from build123d import *

# Parameters (mm, degrees)
SKETCH_1_R          = 1.6
EXTRUDE_1_DEPTH     = 3
CUT_EXTRUDE_1_DEPTH = 85.905830189
FILLET_1_R          = 3
FILLET_2_R          = 10


with BuildPart() as part:
    # 草图1 → 凸台-拉伸1 (new body)
    with BuildSketch(Plane.XY):
        Polygon((0, 0), (20, 0), (60, -40), (60, -60), (0, -60), align=None)
        with Locations((10, -5)):
            Circle(SKETCH_1_R, mode=Mode.SUBTRACT)
        with Locations((10, -25)):
            Circle(SKETCH_1_R, mode=Mode.SUBTRACT)
        with Locations((55, -55)):
            Circle(SKETCH_1_R, mode=Mode.SUBTRACT)
        with Locations(Location((55, -45, 0), (0, 0, 180))):
            Circle(SKETCH_1_R, mode=Mode.SUBTRACT)
        with Locations(Location((45, -55, 0), (0, 0, 180))):
            Circle(SKETCH_1_R, mode=Mode.SUBTRACT)
        with Locations((45, -45)):
            Circle(SKETCH_1_R, mode=Mode.SUBTRACT)
    extrude(amount=EXTRUDE_1_DEPTH)

    # 草图2 → 切除-拉伸1 (cut, through all)
    with BuildSketch(Plane.XY.offset(3)):
        Polygon((40, -60), (0, -60), (0, -30), (20, -30), align=None)
    extrude(amount=-CUT_EXTRUDE_1_DEPTH, mode=Mode.SUBTRACT)

    # 圆角1
    fillet_1_edges = [part.edges().sort_by_distance(p)[0] for p in [
        (0, -30, 1.5),
        (0, 0, 1.5),
        (20, 0, 1.5),
        (60, -40, 1.5),
        (60, -60, 1.5),
    ]]
    fillet(fillet_1_edges, radius=FILLET_1_R)

    # 圆角2
    fillet_2_edges = [part.edges().sort_by_distance(p)[0] for p in [
        (20, -30, 1.5),
    ]]
    fillet(fillet_2_edges, radius=FILLET_2_R)


solid = part.part
CAD build for the part. Positions are in the model's coordinates, mm. A direction names the side the tool comes from. Round coordinates to 2 decimals unless told otherwise and drop trailing zeros. Order: outer loops, then holes, each group sorted by start corner. A loop starts at its lowest first (then second) coordinate and runs counter-clockwise, first axis right, second up. Notation, with made-up numbers: (69.5, 27.5) -> (107.5, 27.5) arc R22 ccw to (107.5, 35.5) -> close; hole circle Ø2 at (32.25, 88). An arc over 180 degrees is marked (long way). Write item = value, one per line. Start each with the question number.
(1) Probe line 1 (Y direction, x = 10, z = 1.9); line 2 (Y direction, x = 55, z = 0.6); line 3 (X direction, y = -56, z = 1.5). List the from-to ranges inside material, lowest first. Write a range as [from, to].
(2) Pull direction X, two halves, no side cores. Call faces 3 (the flat face through (40, -20, 1)), 4 (the cylindrical face through (53.52, -44.39, 1.48)), 5 (the cylindrical face through (44.26, -53.58, 1.48)), 6 (the flat face through (30, -30, 0)): released by +X, released by -X, zero draft, split by the parting line, or undercut.
(3) Cut at C-C, the plane z = 0.7. List the corners of the cut face in (x, y).
(4) Pin check, flat tips, straight feed: P1, Ø1.5, axis at x = 19.5, z = 2.5, coming from the -Y side; P2, Ø3, axis at x = 45, y = -45, coming from the -Z side; P3, Ø1, axis at x = 18.5, z = 1, coming from the -Y side; P4, Ø1.5, axis at x = 7.5, z = 2, coming from the -Y side. Stop position of each tip, or through.
(5) Cut at B-B, the plane y = -45. List the corners of the cut face in (x, z).
(6) Cut at D-D, the plane y = -25. List the corners of the cut face in (x, z).
(7) Which spindle directions (+Z, -Z, +X, -X, +Y, -Y) get a long thin tool onto all of the face, cutting with end or side? Do faces 1 (the flat face through (49, -60, 1)), 2 (the flat face through (9, -30, 2)). Say none if no direction does.
(8) Cut at A-A, the plane x = 10. List the corners of the cut face in (y, z).
Model answer:
q1.line_1 = [-30, -26.6], [-23.4, -6.6], [-3.4, 0]
q1.line_2 = [-60, -56.6], [-53.4, -46.6], [-43.4, -35]
q1.line_3 = [37.33, 43.75], [46.25, 53.75], [56.25, 60]
q2.face_3 = released by +X
q2.face_4 = undercut
q2.face_5 = undercut
q2.face_6 = zero draft
q3.outline = (0, -27) arc R3 ccw to (3, -30) -> (14.65, -30) arc R10 cw to (22.97, -34.45) -> (40, -60) -> (57, -60) arc R3 ccw to (60, -57) -> (60, -41.24) arc R3 ccw to (59.12, -39.12) -> (20.88, -0.88) arc R3 ccw to (18.76, 0) -> (3, 0) arc R3 ccw to (0, -3) -> close; hole circle Ø3.2 at (10, -25); hole circle Ø3.2 at (10, -5); hole circle Ø3.2 at (45, -55); hole circle Ø3.2 at (45, -45); hole circle Ø3.2 at (55, -55); hole circle Ø3.2 at (55, -45)
q4.P1 = -31.72
q4.P2 = through
q4.P3 = -31
q4.P4 = -30
q5.outline = (30, 0) -> (43.4, 0) -> (43.4, 3) -> (30, 3) -> close; (46.6, 0) -> (53.4, 0) -> (53.4, 3) -> (46.6, 3) -> close; (56.6, 0) -> (60, 0) -> (60, 3) -> (56.6, 3) -> close
q6.outline = (0, 0) -> (8.4, 0) -> (8.4, 3) -> (0, 3) -> close; (11.6, 0) -> (45, 0) -> (45, 3) -> (11.6, 3) -> close
q7.face_1 = +Z, -Z, +X, -X, -Y
q7.face_2 = +Z, -Z, -X, -Y
q8.outline = (-30, 0) -> (-26.6, 0) -> (-26.6, 3) -> (-30, 3) -> close; (-23.4, 0) -> (-6.6, 0) -> (-6.6, 3) -> (-23.4, 3) -> close; (-3.4, 0) -> (0, 0) -> (0, 3) -> (-3.4, 3) -> close
